Can you work these out from the drawing? Everything is in mm from the part's minimum corner. Coordinates: 2 decimals unless noted, no trailing zeros. Loops run counter-clockwise (first coordinate to the right, second up) from the corner with the lowest first, then second, coordinate; pieces in that order, holes last.
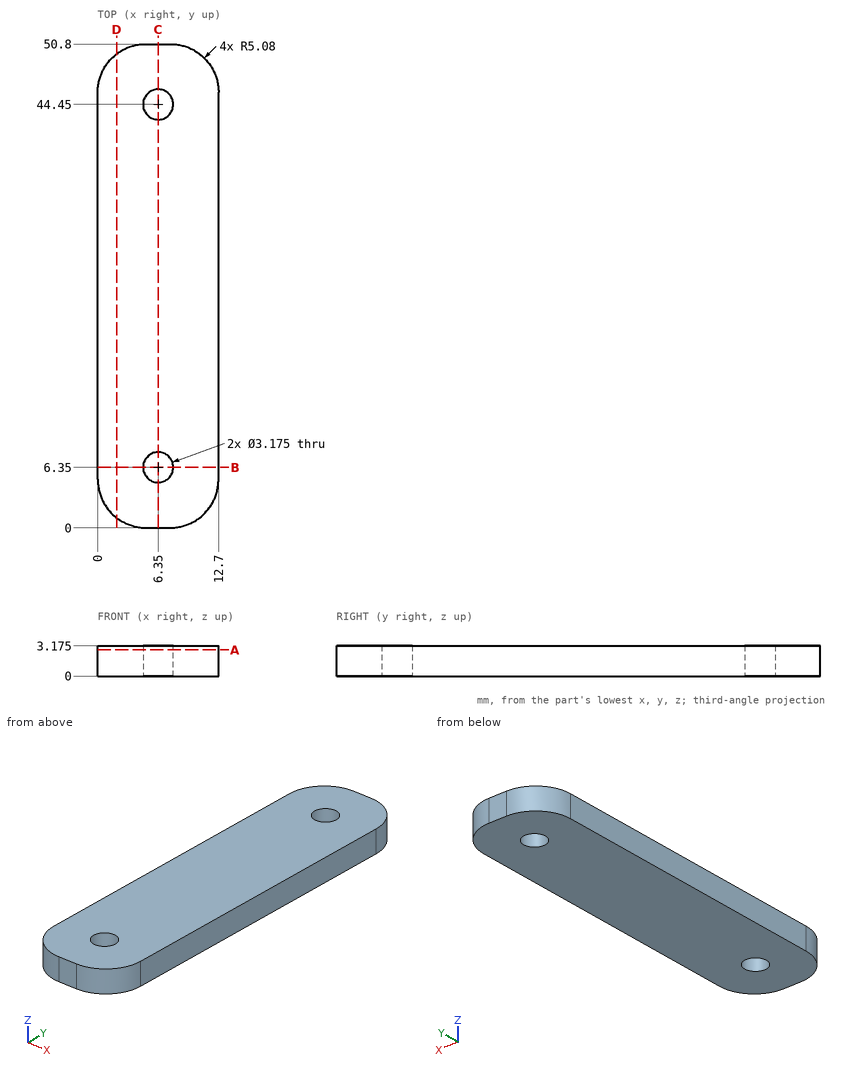
1. I want a section at C-C (x = 6.35). Please give me the cut outline in (y, z) (1 decimal), then the cut area to 3 significant figures.
2. For pin 1 (1 mm diameter, centred on x = 9, z = 1, fed in from +Y), with a flat end and sliding along its axis, tell me the tip position at first contact or that it passes through.
3. I want a section at A-A (z = 2.75). Give the number of separate pieces and of enclosed holes in the cut face, then the cut area to 3 significant figures.
4. I want a section at B-B (y = 6.35). Please give me the cut outline in (x, z) (1 decimal), then the cut area to 3 significant figures.
5. I want a section at D-D (x = 2). Please give me the cut outline in (y, z) (3 decimals), then the cut area to 3 significant figures.
6. I need wall thicknesses on line 1 along Y through (x, z) = (6.35, 0.9); line 2 along X through (y, z) = (3, 2.5); line 3 along Y through (x, z) = (11.75, 0.8). Which ranges of each line are inside material? Lowest first, please.
Response values:
1. outline: (0, 0) - (4.8, 0) - (4.8, 3.2) - (0, 3.2) - close; (7.9, 0) - (42.9, 0) - (42.9, 3.2) - (7.9, 3.2) - close; (46, 0) - (50.8, 0) - (50.8, 3.2) - (46, 3.2) - close
1. area: 141 mm2
2. pin 1: stops at y = 50.72
3. separate pieces: 1
3. enclosed holes: 2
3. area: 607 mm2
4. outline: (0, 0) - (4.8, 0) - (4.8, 3.2) - (0, 3.2) - close; (7.9, 0) - (12.7, 0) - (12.7, 3.2) - (7.9, 3.2) - close
4. area: 30.2 mm2
5. outline: (1.04, 0) - (49.76, 0) - (49.76, 3.175) - (1.04, 3.175) - close
5. area: 155 mm2
6. line 1: y = 0 to 4.76, 7.94 to 42.86, 46.04 to 50.8
6. line 2: x = 0.45 to 12.25
6. line 3: y = 2.12 to 48.68
